Geometry: see drawing. Coordinates: mm, zero at the bounding-box minimum. A direction names the side the tool comes from. Coordinates: 2 decimals unless noted, no trailing zeros. Loops run counter-clockwise (first coordinate to the right, second up) from the corner with the lowest first, then second, coordinate; pieces in that order, holes last. Notation, with made-up numbers: (6.5, -6) - (45.5, -6) arc R25 ccw to (45.5, 20) - close; hole circle Ø2 at (70, 34). An arc over 180 degrees is marked (long way). Answer in a Markdown table with one row per item.
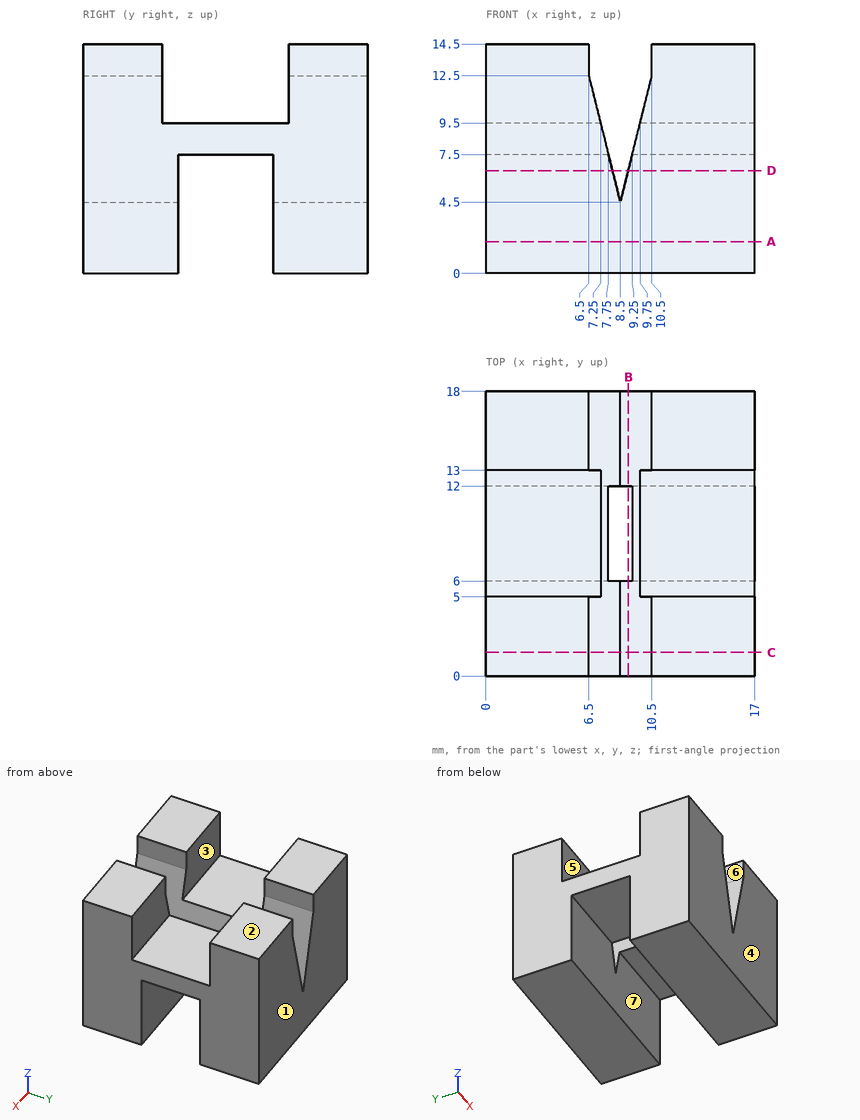
(1) Access query for the marked faces 5, 6 and 7. Directions: +Z, -Z, +X, -X, +Y, -Y. A direction counts if a zero-diameter tool reaches every point of the face in a straight line with its end or side. Return the directions, or none.
Verdict:
| item | result |
|---|---|
| face 5 | +Z, +X, -X |
| face 6 | +Z, +Y, -Y |
| face 7 | -Z, +X, -X |
(2) Pull-direction query (Y, two-part tool) for the marked faces 1, 2, 3 and 4; classes: pulls with the +Y half, pulls with the -Y half, needs draft (parallel to the pull), parting line crosses it, or undercut.
Verdict:
| item | result |
|---|---|
| face 1 | pulls with the +Y half |
| face 2 | needs draft |
| face 3 | undercut |
| face 4 | pulls with the -Y half |
(3) First-contact query: pin 1 Ø5 at (x, y) = (2.5, 9) entering from -Z; pin 2 Ø3.5 at (x, y) = (13, 10) entering from +Z. Flat tips, straight axial feed; report the tip coordinate or a pass-through.
Verdict:
| item | result |
|---|---|
| pin 1 | stops at z = 7.5 |
| pin 2 | stops at z = 9.5 |
(4) Cut plane B-B on x = 9. Output: boundary loops of the cut face in (y, z).
Verdict:
| item | result |
|---|---|
| outline | (0, 0) - (6, 0) - (6, 6.5) - (0, 6.5) - close; (12, 0) - (18, 0) - (18, 6.5) - (12, 6.5) - close |
(5) Cut plane C-C on y = 1.5. Output: boundary loops of the cut face in (x, z).
Verdict:
| item | result |
|---|---|
| outline | (0, 0) - (17, 0) - (17, 14.5) - (10.5, 14.5) - (10.5, 12.5) - (8.5, 4.5) - (6.5, 12.5) - (6.5, 14.5) - (0, 14.5) - close |
(6) Cut plane D-D on z = 6.5. Output: boundary loops of the cut face in (x, y).
Verdict:
| item | result |
|---|---|
| outline | (0, 0) - (8, 0) - (8, 6) - (0, 6) - close; (0, 12) - (8, 12) - (8, 18) - (0, 18) - close; (9, 0) - (17, 0) - (17, 6) - (9, 6) - close; (9, 12) - (17, 12) - (17, 18) - (9, 18) - close |
(7) Cut plane A-A on z = 2. Output: boundary loops of the cut face in (x, y), then the cut area to 3 significant figures.
Verdict:
| item | result |
|---|---|
| outline | (0, 0) - (17, 0) - (17, 6) - (0, 6) - close; (0, 12) - (17, 12) - (17, 18) - (0, 18) - close |
| area | 204 mm² |
(8) Ray query, probe 1 along X at (y, z) = (3, 12.75); probe 2 along Y at (x, z) = (15.5, 0.5); probe 3 along Y at (x, z) = (3.5, 11). Return the intervals inside material, ascending.
Verdict:
| item | result |
|---|---|
| probe 1 | x = 0 to 6.5, 10.5 to 17 |
| probe 2 | y = 0 to 6, 12 to 18 |
| probe 3 | y = 0 to 5, 13 to 18 |
